Autodesk Inventor part; units mm, degrees
ref_plane "YZ Plane" through (0, 0, 0) normal (1, 0, 0) x (0, 1, 0)
ref_plane "XZ Plane" through (0, 0, 0) normal (0, 1, 0) x (-1, 0, 0)
ref_plane "XY Plane" through (0, 0, 0) normal (0, 0, 1) x (1, 0, 0)
sketch "スケッチ1" plane through (0, 0, 0) normal (0, 1, 0) x (-1, 0, 0)
  line L0 (0, -331.5666) -> (0, 61.0944)
  line L1 (-9.0498, 0) -> (7.3416, 0)
  circle A0 centre (0, 0) radius 5
  circle A1 centre (0, 0) radius 3
  arc A2 (4, -267) -> (0, -275) centre (0, -270) ccw
  line L2 (4, -267) -> (4, -3)
  line L3 (-4, -267) -> (-4, -3)
  line L4 (0, -275) -> (0, -265)
  line L5 (4, -267) -> (-4, -267)
  dimension "d0" = 10
  dimension "d1" = 6
  dimension "d2" = 10
  dimension "d3" = 270
  dimension "d4" = 8
extrude "押し出し1" add sketch "スケッチ1" along normal mid plane 10 contours A0 L1 A1 L0 | L0 A1 L1 A0 | A0 L0 A1 L1 | L1 A1 L0 A0
revolve "回転1" add sketch "スケッチ1" angle 360 about axis through (0, 0, 0) along (0, 0, 1) picked at (-0.4059, -272.2831) picked at (-2.4012, -266.7204) contours A2 L5 L0 | L5 A2 L0
extrude "押し出し2" add sketch "スケッチ1" along normal mid plane 8 contours L5 A2 L0 | L0 A2 L5 | L3 A0 L0 A2 | L0 A0 L2 A2 picked at (-2.4012, -266.7204) picked at (2.4012, -266.7204)
properties part number "LinkRod"
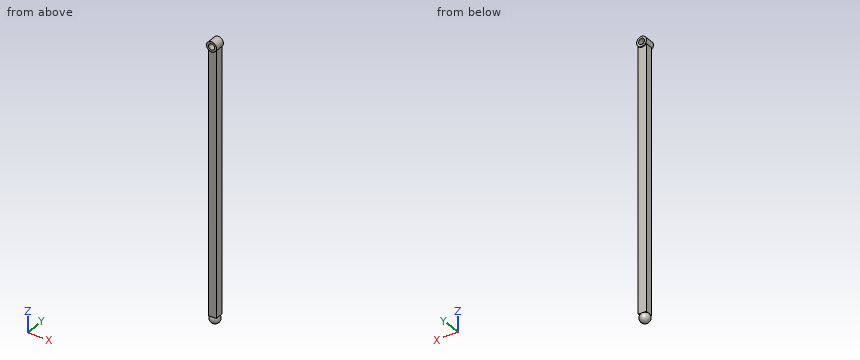
CAD build for the part. Positions are in the model's coordinates, mm. Round coordinates to 2 decimals unless told otherwise and drop trailing zeros. Order: outer loops, then holes, each group sorted by start corner. A loop starts at its lowest first (then second) coordinate and runs counter-clockwise, first axis right, second up.
Q1. Slice it at B-B (z = -248). Write the cut outline in (x, y), and give its area (3 significant figures).
Q2. Slice it at A-A (z = 0). Write the cut outline in (x, y), and give its area (3 significant figures).
Q3. Wall check: L1, parallel to X at y = 2.25, z = 0; L2, parallel to X at y = -2.25, z = -139; L3, parallel to Z at x = 0, y = -0.25. Give the ranges that are in metal, low to high.
Q4. Drop flat-ended pins along their axis: pin 1 (2.5 mm diameter, centred on y = -0.5, z = -103, fed in from +X); pin 2 (3 mm diameter, centred on x = 3, y = 2.5, fed in from -Z); pin 3 (1 mm diameter, centred on x = 3, z = -244.5, fed in from -Y); pin 4 (6 mm diameter, centred on x = 1.5, y = -1.5, fed in from -Z). Give the stop position or say it passes through.
Results below:
1. outline: (-4, -4) - (4, -4) - (4, 4) - (-4, 4) - close
1. area: 64.0 mm2
2. outline: (-5, -5) - (-3, -5) - (-3, 5) - (-5, 5) - close; (3, -5) - (5, -5) - (5, 5) - (3, 5) - close
2. area: 40.0 mm2
3. L1: x = -5 to -3, 3 to 5
3. L2: x = -4 to 4
3. L3: z = -274.99 to -3, 3 to 5
4. pin 1: stops at x = 4
4. pin 2: stops at z = -274.38
4. pin 3: stops at y = -4
4. pin 4: stops at z = -275
